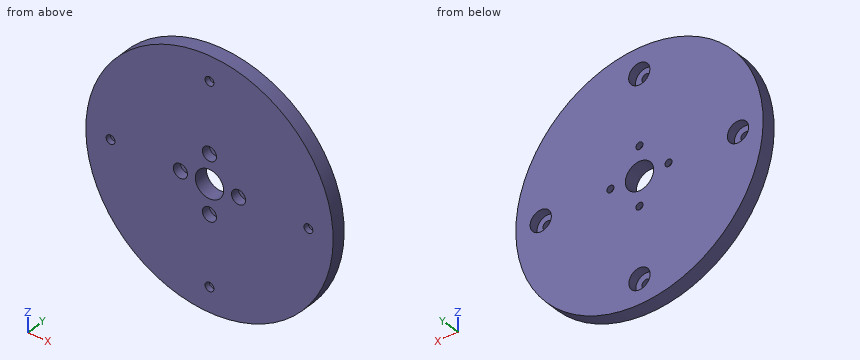
```python
from build123d import *

# Parameters (mm, degrees)
SKETCH1_R           = 35
BOSS_EXTRUDE1_DEPTH = 4
SKETCH2_R           = 1
SKETCH2_R_2         = 1.25
CUT_EXTRUDE1_DEPTH  = 50.658836072
CUT_EXTRUDE2_REACH  = 51.659
SKETCH3_R           = 4
SKETCH4_R           = 3
CUT_EXTRUDE3_DEPTH  = 2.5
SKETCH5_R           = 2
CUT_EXTRUDE4_DEPTH  = 2.5


with BuildPart() as part:
    # Sketch1 → Boss-Extrude1 (new body)
    with BuildSketch(Plane(origin=(0, 0, 0), x_dir=(1, 0, 0), z_dir=(0, 1, 0))):
        with Locations(Location((0, 0, 0), (0, 0, 270))):
            Circle(SKETCH1_R)
    extrude(amount=BOSS_EXTRUDE1_DEPTH)

    # Sketch2 → Cut-Extrude1 (cut, through all)
    with BuildSketch(Plane(origin=(0, 4, 0), x_dir=(1, 0, 0), z_dir=(0, 1, 0))):
        with Locations(Location((0, 8.227062517, 0), (0, 0, 270))):
            Circle(SKETCH2_R)
        with Locations(Location((8.227062517, 0, 0), (0, 0, 270))):
            Circle(SKETCH2_R)
        with Locations(Location((0, -8.227062517, 0), (0, 0, 270))):
            Circle(SKETCH2_R)
        with Locations(Location((-8.227062517, 0, 0), (0, 0, 270))):
            Circle(SKETCH2_R)
        with Locations(Location((0, -28, 0), (0, 0, 90))):
            Circle(SKETCH2_R_2)
        with Locations(Location((-28, 0, 0), (0, 0, 90))):
            Circle(SKETCH2_R_2)
        with Locations(Location((0, 28, 0), (0, 0, 90))):
            Circle(SKETCH2_R_2)
        with Locations(Location((28, 0, 0), (0, 0, 90))):
            Circle(SKETCH2_R_2)
    extrude(amount=-CUT_EXTRUDE1_DEPTH, mode=Mode.SUBTRACT)

    # Sketch3 → Cut-Extrude2 (cut, up to next)
    with BuildSketch(Plane.XZ, mode=Mode.PRIVATE) as cut_extrude2_sk1:
        with Locations(Location((0, 0, 0), (0, 0, 270))):
            Circle(SKETCH3_R)
    cut_extrude2_tool1 = extrude(cut_extrude2_sk1.sketch, amount=-CUT_EXTRUDE2_REACH, mode=Mode.PRIVATE) & part.part
    add(cut_extrude2_tool1.solids().sort_by_distance((0, 0, 0))[0], mode=Mode.SUBTRACT)

    # Sketch4 → Cut-Extrude3 (cut)
    with BuildSketch(Plane(origin=(0, 4, 0), x_dir=(1, 0, 0), z_dir=(0, 1, 0))):
        with Locations(Location((0, 28, 0), (0, 0, 270))):
            Circle(SKETCH4_R)
        with Locations(Location((27.948073418, 0.109503391, 0), (0, 0, 270))):
            Circle(SKETCH4_R)
        with Locations(Location((0.057576809, -27.838570027, 0), (0, 0, 270))):
            Circle(SKETCH4_R)
        with Locations(Location((-27.890496609, 0.051926582, 0), (0, 0, 270))):
            Circle(SKETCH4_R)
    extrude(amount=-CUT_EXTRUDE3_DEPTH, mode=Mode.SUBTRACT)

    # Sketch5 → Cut-Extrude4 (cut)
    with BuildSketch(Plane.XZ):
        with Locations(Location((0, 8.227062517, 0), (0, 0, 270))):
            Circle(SKETCH5_R)
        with Locations(Location((8.227062517, 0, 0), (0, 0, 270))):
            Circle(SKETCH5_R)
        with Locations(Location((0, -8.227062517, 0), (0, 0, 270))):
            Circle(SKETCH5_R)
        with Locations(Location((-8.227062517, 0, 0), (0, 0, 270))):
            Circle(SKETCH5_R)
    extrude(amount=-CUT_EXTRUDE4_DEPTH, mode=Mode.SUBTRACT)


solid = part.part
```
Work out the finished part from the listing and answer in its coordinate system (mm). Coordinates: 2 decimals unless noted, no trailing zeros. Write each loop counter-clockwise with the first axis right and the second up, starting at its lowest first coordinate (ties: lowest second). Pieces come first, ordered by that corner, then holes.
Q1. Each of these flat-tipped pins is pushed along its axis until it touches: pin 1 Ø2 at (x, z) = (-9, -0.5) entering from -Y; pin 2 Ø1 at (y, z) = (2.5, -19) entering from -X; pin 3 Ø3 at (x, z) = (-28, 0) entering from +Y. Where does it stop, or does it pass through?
Q2. A cutting plane is placed at D-D, the plane z = 11.5. Give the vertices of the cut face in (x, y).
Q3. A cutting plane is placed at C-C, the plane x = 11.5. Give the vertices of the cut face in (y, z), then the cut area to 3 significant figures.
Q4. Find the intervals of material crossed by line 1 (X direction, y = 0.9, z = 0); line 2 (X direction, y = 1.8, z = 0); line 3 (Y direction, x = -28, z = 2.5), in increasing order.
Q5. A cutting plane is placed at B-B, the plane z = 0. State how many separate pieces and enclosed holes the cut face has, then the cut area to 3 significant figures.
Q6. A cutting plane is placed at A-A, the plane z = -28. Give the vertices of the cut face in (x, y), then the cut area to 3 significant figures.
Findings below:
1. pin 1: stops at y = 2.5
1. pin 2: stops at x = -29.71
1. pin 3: stops at y = 1.5
2. outline: (-33.06, 0) - (33.06, 0) - (33.06, 4) - (-33.06, 4) - close
3. outline: (0, -33.06) - (4, -33.06) - (4, 33.06) - (0, 33.06) - close
3. area: 264 mm2
4. line 1: x = -35 to -29.25, -26.75 to -10.23, -6.23 to -4, 4 to 6.23, 10.23 to 26.75, 29.25 to 35
4. line 2: x = -35 to -30.89, -24.89 to -10.23, -6.23 to -4, 4 to 6.23, 10.23 to 24.95, 30.95 to 35
4. line 3: y = 0 to 1.5
5. separate pieces: 6
5. enclosed holes: 0
5. area: 185 mm2
6. outline: (-21, 0) - (-1.25, 0) - (-1.25, 1.5) - (-3, 1.5) - (-3, 4) - (-21, 4) - close; (1.25, 0) - (21, 0) - (21, 4) - (3, 4) - (3, 1.5) - (1.25, 1.5) - close
6. area: 149 mm2
